Part print with two shaded views. Sizes in mm from the minimum x, y, z corner. Round coordinates to 2 decimals unless told otherwise and drop trailing zeros. Loops run counter-clockwise (first coordinate to the right, second up) from the corner with the lowest first, then second, coordinate; pieces in that order, holes last. Notation, with made-up numbers: M -7.75,64.25 L 6.25,64.25 A15 cw 6.25,77.25 Z; hole C -9.5,45 d9. An arc over 180 degrees is marked long. Put each result on its own line as item: value. Start each with the question number.
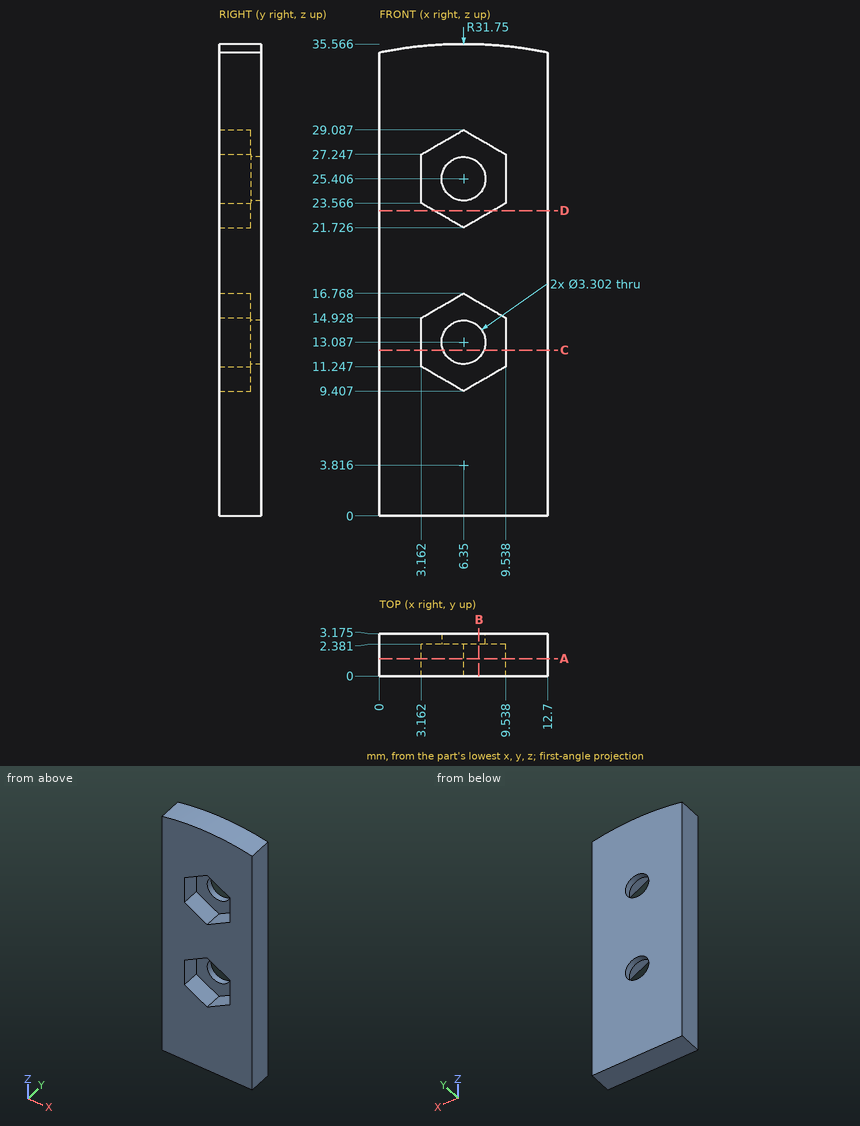
(1) Cut at C-C on z = 12.5. List the corners of the cut face in (x, y) (1 decimal).
(2) Flat gauge pins, fed straight in: pin 1 Ø1.5 at (x, y) = (8.5, 2) entering from +Z; pin 2 Ø1.5 at (x, z) = (4, 14) entering from -Y. Where does each tip first touch, or does it go through?
(3) Cut at B-B on x = 7.5. List the corners of the cut face in (y, z) (1 decimal).
(4) Cut at D-D on z = 23. List the corners of the cut face in (x, y) (1 decimal), and give its area (3 significant figures).
(5) Cut at A-A on y = 1.3. Count the separate pieces of the cut face and the enclosed holes in it.
(6) Drill centre lines: line 1 along Z through (x, y) = (6.35, 2.95) (1 decimal); line 2 along Z through (x, y) = (5.25, 0.35) (1 decimal); line 3 along X through (y, z) = (1.65, 24). Where is each one in solid material? Low to high.
Taken from the geometry:
1. outline: M 0,0 L 3.2,0 L 3.2,2.4 L 4.8,2.4 L 4.8,3.2 L 0,3.2 Z; M 7.9,2.4 L 9.5,2.4 L 9.5,0 L 12.7,0 L 12.7,3.2 L 7.9,3.2 Z
2. pin 1: z = 35.54
2. pin 2: y = 2.38
3. outline: M 0,0 L 3.2,0 L 3.2,11.9 L 2.4,11.9 L 2.4,10.1 L 0,10.1 Z; M 0,16.1 L 2.4,16.1 L 2.4,14.3 L 3.2,14.3 L 3.2,24.2 L 2.4,24.2 L 2.4,22.4 L 0,22.4 Z; M 0,28.4 L 2.4,28.4 L 2.4,26.6 L 3.2,26.6 L 3.2,35.5 L 0,35.5 Z
4. outline: M 0,0 L 4.1,0 L 4.1,2.4 L 8.6,2.4 L 8.6,0 L 12.7,0 L 12.7,3.2 L 0,3.2 Z
4. area: 29.8 mm2
5. separate pieces: 1
5. enclosed holes: 2
6. line 1: 0 to 11.4, 14.7 to 23.8, 27.1 to 35.6
6. line 2: 0 to 10, 16.1 to 22.4, 28.5 to 35.5
6. line 3: 0 to 3.16, 9.54 to 12.7
